Geometry: final body of the model. Coordinates: model frame, mm. A direction names the side the tool comes from. Round coordinates to 2 decimals unless told otherwise and drop trailing zeros. Write each loop counter-clockwise with the first axis right and the second up, starting at its lowest first coordinate (ties: lowest second). Pieces come first, ordered by that corner, then holes. Notation, with made-up numbers: M 38.5,-29.5 L 97.5,-29.5 A20 cw 97.5,-2.5 Z; hole C 15,6.5 d9. An arc over 180 degrees is marked long. Answer as CSV lines item,"result". Start each with the question number.
Q1. Ray query, probe 1 along Y at (x, z) = (-154.5, 131.5); probe 2 along X at (y, z) = (309, 67.5); probe 3 along Z at (x, y) = (-82.5, 283) (3 decimals). Return the intervals inside material, ascending.
Q2. Reachability of faces 1 (the flat face through (32, 390.778, 105)), 2 (the flat face through (516, 327.278, 7)), 3 (the flat face through (457.2, 363, 83)) from +Z, -Z, +X, -X, +Y, -Y: full face, straight path, thin tool, end or side. Return the list, or none.
Q3. Section query C-C on x = -199. Output: boundary loops of the cut face in (y, z) (3 decimals), and give its area (3 significant figures).
Q4. First-contact query: pin 1 (3 mm diameter, centred on x = 460, z = 163.5, fed in from +Y); pin 2 (4 mm diameter, centred on x = 415, y = -361.5, fed in from +Z) (3 decimals); pin 3 (1.9 mm diameter, centred on x = -411, y = -178.5, fed in from +Z). Flat tips, straight axial feed; report the tip coordinate or a pass-through.
Q5. Section query A-A on z = 156.5. Output: boundary loops of the cut face in (x, y).
Q6. Mould query, pull axis X, two halves, no side actions, for faces 4 (the flat face through (19, -390.778, 105)), 5 (the flat face through (463.55, 366, 83)), 6 (the flat face through (16, 384.428, 105)), 7 (the flat face through (-412.75, 5, 83)). Classes: pulls with the +X half, pulls with the -X half, needs draft (parallel to the pull), parting line crosses it, or undercut.
Q7. Section query D-D on z = 32. Output: boundary loops of the cut face in (x, y).
Q8. Section query B-B on y = -95. Output: boundary loops of the cut face in (x, z) (3 decimals).
```python
from build123d import *

# Parameters (mm, degrees)
F0_W     = 6.35
F0_H     = 28.575
F0_H_2   = 31.75
F1_DEPTH = 9.525
F2_DEPTH = 76.2
F3_DEPTH = 203.2
F4_DEPTH = 139.7
F5_DEPTH = 203.2


with BuildPart() as f1:
    # F0 (on Top) → F1 (new body)
    with BuildSketch(Plane.XY):
        Polygon((-609.6, -533.4), (609.6, -533.4), (609.6, -327.277558), (463.55, -327.277558), (463.55, -355.852558), (463.55, -390.777558), (457.2, -390.777558), (-412.75, -390.777558), (-412.75, -384.427558), (-412.75, 0), (-412.75, 384.427558), (-412.75, 390.777558), (457.2, 390.777558), (463.55, 390.777558), (463.55, 359.027558), (463.55, 327.277558), (609.6, 327.277558), (609.6, 533.4), (-609.6, 533.4), (-609.6, 0), align=None)
        with Locations((460.375, -341.565058)):
            Rectangle(F0_W, F0_H)
        Polygon((457.2, -355.852558), (457.2, -327.277558), (457.2, 0), (457.2, 327.277558), (457.2, 359.027558), (457.2, 384.427558), (-406.4, 384.427558), (-406.4, 0), (-406.4, -384.427558), (457.2, -384.427558), align=None)
        with Locations((460.375, 343.152558)):
            Rectangle(F0_W, F0_H_2)
    extrude(amount=F1_DEPTH)

    # F0 (on Top) → F2 (join)
    with BuildSketch(Plane.XY):
        with Locations((460.375, 343.152558)):
            Rectangle(F0_W, F0_H_2)
        with Locations((460.375, -341.565058)):
            Rectangle(F0_W, F0_H)
    extrude(amount=F2_DEPTH)

    # F0 (on Top) → F3 (join)
    with BuildSketch(Plane.XY):
        Polygon((463.55, -390.777558), (463.55, -355.852558), (457.2, -355.852558), (457.2, -384.427558), (-406.4, -384.427558), (-412.75, -384.427558), (-412.75, -390.777558), (457.2, -390.777558), align=None)
    extrude(amount=F3_DEPTH)

    # F0 (on Top) → F4 (join)
    with BuildSketch(Plane.XY):
        Polygon((-412.75, -384.427558), (-406.4, -384.427558), (-406.4, 0), (-406.4, 384.427558), (-412.75, 384.427558), (-412.75, 0), align=None)
    extrude(amount=F4_DEPTH)

    # F0 (on Top) → F5 (join)
    with BuildSketch(Plane.XY):
        Polygon((457.2, 384.427558), (457.2, 359.027558), (463.55, 359.027558), (463.55, 390.777558), (457.2, 390.777558), (-412.75, 390.777558), (-412.75, 384.427558), (-406.4, 384.427558), align=None)
    extrude(amount=F5_DEPTH)


solid = f1.part
```
Entries:
1,probe 1,"y = -390.78 to -384.43, 384.43 to 390.78"
1,probe 2,"x = -412.75 to -406.4"
1,probe 3,"z = 0 to 9.525"
2,face 1,"+Z, +X, -X, +Y"
2,face 2,"+Z, -Z, +X"
2,face 3,"+Z"
3,outline,"M -533.4,0 L 533.4,0 L 533.4,9.525 L 390.778,9.525 L 390.778,203.2 L 384.428,203.2 L 384.428,9.525 L -384.428,9.525 L -384.428,203.2 L -390.778,203.2 L -390.778,9.525 L -533.4,9.525 Z"
3,area,"12,600 mm^2"
4,pin 1,"stops at y = 390.78"
4,pin 2,"stops at z = 9.525"
4,pin 3,"stops at z = 139.7"
5,outline,"M -412.75,-390.78 L 463.55,-390.78 L 463.55,-355.85 L 457.2,-355.85 L 457.2,-384.43 L -412.75,-384.43 Z; M -412.75,384.43 L 457.2,384.43 L 457.2,359.03 L 463.55,359.03 L 463.55,390.78 L -412.75,390.78 Z"
6,face 4,"needs draft"
6,face 5,"pulls with the +X half"
6,face 6,"undercut"
6,face 7,"pulls with the -X half"
7,outline,"M -412.75,-390.78 L 463.55,-390.78 L 463.55,-327.28 L 457.2,-327.28 L 457.2,-384.43 L -406.4,-384.43 L -406.4,384.43 L 457.2,384.43 L 457.2,327.28 L 463.55,327.28 L 463.55,390.78 L -412.75,390.78 Z"
8,outline,"M -609.6,0 L 457.2,0 L 457.2,9.525 L -406.4,9.525 L -406.4,139.7 L -412.75,139.7 L -412.75,9.525 L -609.6,9.525 Z"
